Could you check a few things on this model? Use its own coordinates, in mm. Face numbers are marked on the shaded views. Coordinates: 2 decimals unless noted, no trailing zeros. Loops run counter-clockwise (first coordinate to the right, second up) from the corner with the lowest first, then second, coordinate; pieces in that order, holes last. Notation, with made-up numbers: (70, -25) -> (83, -25) arc R27 ccw to (83, 14) -> close; hole circle Ø1 at (82, 1.25). An arc over 180 degrees is marked (long way). One line per question, with ' | ' between items. Start each with the question number.
(1) I'm going to push flat-ended pins straight in: pin 1 Ø2 at (x, y) = (-3, 16.5) entering from +Z; pin 2 Ø2 at (x, y) = (-3, 16.5) entering from -Z; pin 3 Ø3 at (x, y) = (-3, -16.5) entering from +Z; pin 4 Ø3 at (y, z) = (-13.5, 5.5) entering from -X. Where does each tip first touch, or does it pass through?
(2) Suppose I cut it at D-D (y = 11). Please give me the cut outline in (x, z), plus the area to 3 significant figures.
(3) If I drill on line 1 along Y through (x, z) = (-2.5, 3.75); line 2 along Y through (x, z) = (-3, 18.5); line 3 along X through (y, z) = (17.5, 5.5), over which ranges is the centre line in solid material (lowest first)?
(4) Suppose I cut it at C-C (z = 11). Please give me the cut outline in (x, y), plus the area to 3 significant figures.
(5) Suppose I cut it at B-B (x = -7). Please give me the cut outline in (y, z), plus the area to 3 significant figures.
(6) If we mould it in two halves opening along Y, with no side actions, what happens to the marked faces 1, 2 and 3? For each: pulls with the +Y half, pulls with the -Y half, needs draft (parallel to the pull), parting line crosses it, or undercut.
(7) Suppose I cut it at A-A (z = 19.5). Please give me the cut outline in (x, y).
```python
from build123d import *

# Parameters (mm, degrees)
SKETCH_1_W                       = 8.5
SKETCH_1_H                       = 39
EXTRUDE_1_DEPTH                  = 22.3
SKETCH_2_R                       = 22
CUT_EXTRUDE_2_DEPTH              = 22.3
HOLE_WIZARD_M3_1_D               = 2.5
HOLE_WIZARD_M3_1_DEPTH           = 9.5
HOLE_WIZARD_M3_1_TIP             = 0.751075774
HOLE_WIZARD_M3_2_D               = 2.5
HOLE_WIZARD_M3_2_DEPTH           = 9.5
HOLE_WIZARD_M3_2_TIP             = 0.751075774
HOLE_WIZARD_M3_3_D               = 2.5
HOLE_WIZARD_M3_3_DEPTH           = 9.5
HOLE_WIZARD_M3_3_TIP             = 0.751075774
HOLE_WIZARD_M3_3_ON_FACE_2_D     = 2.5
HOLE_WIZARD_M3_3_ON_FACE_2_DEPTH = 9.5
HOLE_WIZARD_M3_3_ON_FACE_2_TIP   = 0.751075774
CHAMFER_2_SIZE                   = 6
CHAMFER_2_SIZE_2                 = 2.797845949
CHAMFER_5_SIZE                   = 2.797845949
CHAMFER_5_SIZE_2                 = 6
EXTRUDE_5_DEPTH                  = 39


with BuildPart() as part:
    # 草图1 → 拉伸1 (new body)
    with BuildSketch(Plane.XY):
        with Locations((-4.25, 0)):
            Rectangle(SKETCH_1_W, SKETCH_1_H)
    extrude(amount=EXTRUDE_1_DEPTH)

    # 草图2 → 拉伸2 (cut)
    with BuildSketch(Plane.XY.offset(22.3)):
        with Locations((14.5, 0)):
            Circle(SKETCH_2_R)
    extrude(amount=-CUT_EXTRUDE_2_DEPTH, mode=Mode.SUBTRACT)

    # M3 螺纹孔1
    with Locations(Plane(origin=(-3, 16.5, 22.3), x_dir=(1, 0, 0), z_dir=(0, 0, 1))):
        with Locations((0, 0)):
            Hole(HOLE_WIZARD_M3_1_D / 2, depth=HOLE_WIZARD_M3_1_DEPTH)
            with Locations((0, 0, -(HOLE_WIZARD_M3_1_DEPTH + HOLE_WIZARD_M3_1_TIP / 2))):  # 118° drill point
                Cone(0, HOLE_WIZARD_M3_1_D / 2, HOLE_WIZARD_M3_1_TIP, mode=Mode.SUBTRACT)

    # M3 螺纹孔2
    with Locations(Plane(origin=(-3, 16.5, 0), x_dir=(-1, 0, 0), z_dir=(0, 0, -1))):
        with Locations((0, 0)):
            Hole(HOLE_WIZARD_M3_2_D / 2, depth=HOLE_WIZARD_M3_2_DEPTH)
            with Locations((0, 0, -(HOLE_WIZARD_M3_2_DEPTH + HOLE_WIZARD_M3_2_TIP / 2))):  # 118° drill point
                Cone(0, HOLE_WIZARD_M3_2_D / 2, HOLE_WIZARD_M3_2_TIP, mode=Mode.SUBTRACT)

    # M3 螺纹孔3
    with Locations(Plane(origin=(-3, -16.5, 22.3), x_dir=(1, 0, 0), z_dir=(0, 0, 1))):
        with Locations((0, 0)):
            Hole(HOLE_WIZARD_M3_3_D / 2, depth=HOLE_WIZARD_M3_3_DEPTH)
            with Locations((0, 0, -(HOLE_WIZARD_M3_3_DEPTH + HOLE_WIZARD_M3_3_TIP / 2))):  # 118° drill point
                Cone(0, HOLE_WIZARD_M3_3_D / 2, HOLE_WIZARD_M3_3_TIP, mode=Mode.SUBTRACT)

    # M3 螺纹孔3 on face 2
    with Locations(Plane(origin=(-3, -16.5, 0), x_dir=(-1, 0, 0), z_dir=(0, 0, -1))):
        with Locations((0, 0)):
            Hole(HOLE_WIZARD_M3_3_ON_FACE_2_D / 2, depth=HOLE_WIZARD_M3_3_ON_FACE_2_DEPTH)
            with Locations((0, 0, -(HOLE_WIZARD_M3_3_ON_FACE_2_DEPTH + HOLE_WIZARD_M3_3_ON_FACE_2_TIP / 2))):  # 118° drill point
                Cone(0, HOLE_WIZARD_M3_3_ON_FACE_2_D / 2, HOLE_WIZARD_M3_3_ON_FACE_2_TIP, mode=Mode.SUBTRACT)

    # 倒角2
    # the kernel refuses this chamfer: 6, 2.797845949 mm, written as the material it takes off along each edge
    with BuildSketch(Plane(origin=(-8.5, -35.045852829, 22.3), x_dir=(-0.01631116413111048, 0, -0.9998669641130704), z_dir=(0, 1, 0))) as chamfer_2_piece_1:
        Polygon((CHAMFER_2_SIZE * 0.999866964113, -CHAMFER_2_SIZE * 0.0163111641311), (-CHAMFER_2_SIZE_2 * 0.0163111641307, -CHAMFER_2_SIZE_2 * 0.999866964088), (0, 0), align=None)
    extrude(amount=70.091705657, mode=Mode.SUBTRACT)

    # 倒角5
    # the kernel refuses this chamfer: 6, 2.797845949 mm, written as the material it takes off along each edge
    with BuildSketch(Plane(origin=(-8.5, -35.045852829, 0), x_dir=(0.9971975577536775, 0, -0.07481330637059953), z_dir=(0, 1, 0))) as chamfer_5_piece_1:
        Polygon((CHAMFER_5_SIZE * 0.997197557729, -CHAMFER_5_SIZE * 0.0748133063687), (-CHAMFER_5_SIZE_2 * 0.0748133063706, -CHAMFER_5_SIZE_2 * 0.997197557754), (0, 0), align=None)
    extrude(amount=70.091705657, mode=Mode.SUBTRACT)

    # 草图8 → 拉伸5 (add)
    with BuildSketch(Plane(origin=(0, 19.5, 0), x_dir=(1, 0, 0), z_dir=(0, 1, 0))):
        Polygon((-8.5, -16.3), (-8.5, -6), (-9, -7.07225346), (-9, -15.22774654), align=None)
    extrude(amount=-EXTRUDE_5_DEPTH)


solid = part.part
```
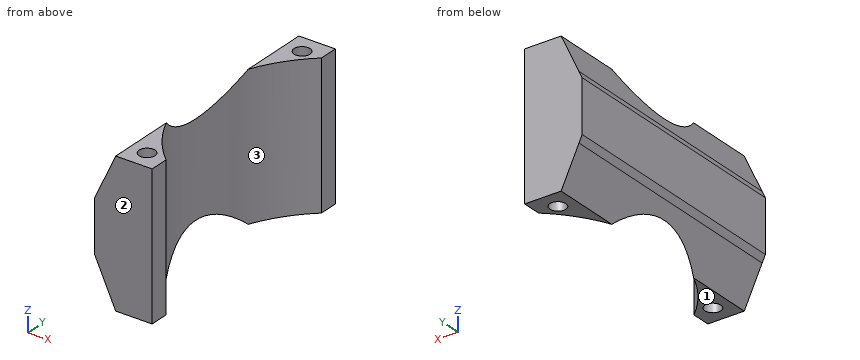
Checks:
1) pin 1: stops at z = 12.65 | pin 2: stops at z = 9.65 | pin 3: stops at z = 22.3 | pin 4: stops at x = -8.97
2) outline: (-9, 7.07) -> (-5.7, 0) -> (-4.55, 0) -> (-4.55, 22.3) -> (-5.7, 22.3) -> (-9, 15.23) -> close | area: 75.9 mm^2
3) line 1: y = -19.5 to -17.65, -15.35 to -13.96, 13.96 to 15.35, 17.65 to 19.5 | line 2: y = -19.5 to -17.75, -15.25 to -13.33, 13.33 to 15.25, 17.75 to 19.5 | line 3: x = -8.27 to -3.75, -2.25 to 0
4) outline: (-9, -19.5) -> (0, -19.5) -> (0, -16.55) arc R22 cw to (0, 16.55) -> (0, 19.5) -> (-9, 19.5) -> close | area: 179 mm^2
5) outline: (-19.5, 2.78) -> (-4.66, 2.78) -> (-4.66, 19.52) -> (-19.5, 19.52) -> close; (4.66, 2.78) -> (19.5, 2.78) -> (19.5, 19.52) -> (4.66, 19.52) -> close | area: 497 mm^2
6) face 1: needs draft | face 2: pulls with the -Y half | face 3: undercut
7) outline: (-7.01, -19.5) -> (0, -19.5) -> (0, -16.55) arc R22 cw to (-7.01, -4.63) -> close; (-7.01, 4.63) arc R22 cw to (0, 16.55) -> (0, 19.5) -> (-7.01, 19.5) -> close; hole circle Ø2.5 at (-3, -16.5); hole circle Ø2.5 at (-3, 16.5)
